Source: CAD feature listing. Evaluate the final solid. Frame: model axes, mm. Face numbers are marked on the shaded views. A direction names the side the tool comes from. Give positions to 0.01 mm unless a question says otherwise; leave off trailing zeros. Order: outer loops, then holes, each group sorted by start corner. A loop starts at its lowest first (then second) coordinate and runs counter-clockwise, first axis right, second up. Notation, with made-up numbers: M 24,40 L 58,40 A14 cw 58,60 Z; hole C 66.25,88 d7. An arc over 180 degrees is marked long. Return JSON: item names as keys, results as strings.
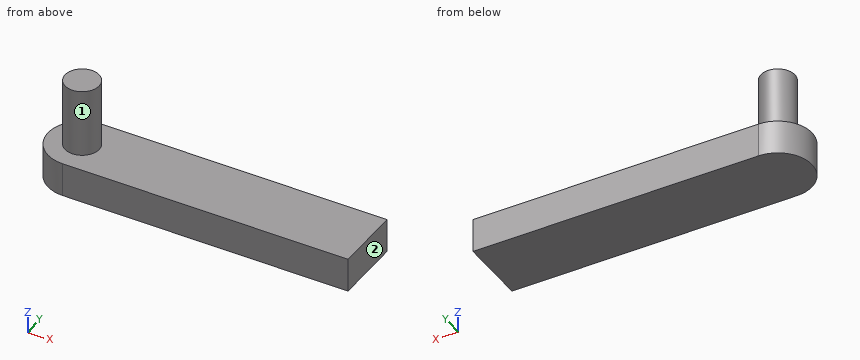
from build123d import *

# Parameters (mm, degrees)
SKETCH1_R                = 2.5
BOSS_EXTRUDE1_DEPTH      = 10
SKETCH2_R                = 5
BOSS_EXTRUDE2_DEPTH      = 5
BOSS_EXTRUDE3_REACH      = 20.708
BOSS_EXTRUDE3_END_RADIUS = 5
SKETCH4_W                = 5
SKETCH4_H                = 10
SKETCH5_W                = 5
SKETCH5_H                = 10
BOSS_EXTRUDE4_DEPTH      = 32


with BuildPart() as part:
    # Sketch1 → Boss-Extrude1 (new body)
    with BuildSketch(Plane.XY):
        Circle(SKETCH1_R)
    extrude(amount=BOSS_EXTRUDE1_DEPTH)

    # Sketch2 → Boss-Extrude2 (add)
    with BuildSketch(Plane(origin=(0, 0, 0), x_dir=(-1, 0, 0), z_dir=(0, 0, -1))):
        Circle(SKETCH2_R)
    extrude(amount=BOSS_EXTRUDE2_DEPTH)

    # Boss-Extrude3: up to this cylinder (the profile starts outside it)
    boss_extrude3_end = Plane(origin=(0, 0, -2.5), z_dir=(0, 0, 1)) * Cylinder(BOSS_EXTRUDE3_END_RADIUS, 52.416, mode=Mode.PRIVATE)
    # Sketch4 → Boss-Extrude3 (add, up to the surface)
    with BuildSketch(Plane(origin=(10, 0, 0), x_dir=(0, 0, -1), z_dir=(1, 0, 0)), mode=Mode.PRIVATE) as boss_extrude3_sk1:
        with Locations((2.5, 0)):
            Rectangle(SKETCH4_W, SKETCH4_H)
    boss_extrude3_tool1 = extrude(boss_extrude3_sk1.sketch, amount=-BOSS_EXTRUDE3_REACH, mode=Mode.PRIVATE) - boss_extrude3_end
    add(boss_extrude3_tool1.solids().sort_by_distance((10, 0, -2.5))[0])

    # Sketch5 → Boss-Extrude4 (add)
    with BuildSketch(Plane(origin=(10, 0, 0), x_dir=(0, 0, -1), z_dir=(1, 0, 0))):
        with Locations((2.5, 0)):
            Rectangle(SKETCH5_W, SKETCH5_H)
    extrude(amount=BOSS_EXTRUDE4_DEPTH)


solid = part.part
1. First-contact query: pin 1 (3 mm diameter, centred on x = 27.5, y = -2, fed in from +Z); pin 2 (2 mm diameter, centred on x = 13, z = 0.5, fed in from -Y). Flat tips, straight axial feed; report the tip coordinate or a pass-through.
Evaluation:
{"pin 1": "stops at z = 0", "pin 2": "stops at y = -5"}
2. Section query D-D (x = 23). Return loops of the section in (y, z), then the cut area to 3 significant figures.
Evaluation:
{"outline": "M -5,-5 L 5,-5 L 5,0 L -5,0 Z", "area": "50.0 mm^2"}
3. Section query B-B (z = 7.75). Return loops of the section in (x, y), then the cut area to 3 significant figures.
Evaluation:
{"outline": "C 0,0 d5", "area": "19.6 mm^2"}
4. Set-up query: the marked faces 1 and 2. Return all of +Z, -Z, +X, -X, +Y, -Y with unobstructed straight access to the full face (end or side cutting, diameter ignored); none if empty.
Evaluation:
{"face 1": "+Z", "face 2": "+Z, -Z, +X, +Y, -Y"}
5. Ray query, probe 1 along Z at (x, y) = (34.5, -0.5); probe 2 along X at (y, z) = (0.75, 9.25); probe 3 along Y at (x, z) = (-1, 7.5). Return the intervals inside material, ascending.
Evaluation:
{"probe 1": "z = -5 to 0", "probe 2": "x = -2.38 to 2.38", "probe 3": "y = -2.29 to 2.29"}
6. Section query C-C (x = 1). Return loops of the section in (y, z).
Evaluation:
{"outline": "M -5,-5 L 5,-5 L 5,0 L 2.29,0 L 2.29,10 L -2.29,10 L -2.29,0 L -5,0 Z"}
7. Section query A-A (y = 0). Return loops of the section in (x, z).
Evaluation:
{"outline": "M -5,-5 L 42,-5 L 42,0 L 2.5,0 L 2.5,10 L -2.5,10 L -2.5,0 L -5,0 Z"}
